Model file for the job. Use its own axes, mm. Face numbers are marked on the shaded views. Coordinates: 2 decimals unless noted, no trailing zeros. Write each loop counter-clockwise with the first axis right and the second up, starting at its lowest first coordinate (ties: lowest second). Pieces come first, ordered by that corner, then holes. Notation, with made-up numbers: M -32,74 L 24,74 A18 ccw 24,83 Z; hole C 13,83 d7. An arc over 180 degrees is marked long. Use CSV: the item, a comma, the result in double quotes. Start each with the question number.
from build123d import *

# Parameters (mm, degrees)
SKETCH1_W              = 22.5552
SKETCH1_H              = 12.7
BOSS_EXTRUDE1_DEPTH    = 1
SKETCH2_W              = 5
SKETCH2_H              = 7.3
CUT_EXTRUDE1_DEPTH     = 1
SKETCH3_W              = 5
SKETCH3_H              = 5
CUT_EXTRUDE2_DEPTH     = 1
SKETCH4_W              = 22.0552
SKETCH4_H              = 0.5
SKETCH4_W_2            = 0.5
SKETCH4_H_2            = 1.5
SKETCH4_H_3            = 2
BOSS_EXTRUDE2_DEPTH    = 1
SKETCH5_W              = 39.7552
SKETCH5_H              = 16.7
BOSS_EXTRUDE3_DEPTH    = 1
CUT_EXTRUDE3_DEPTH     = 1
CUT_EXTRUDE4_DEPTH     = 1
CUT_EXTRUDE5_START     = -4
CUT_EXTRUDE5_DEPTH     = 5
SKETCH10_W             = 22.5552
SKETCH10_H             = 2
BOSS_EXTRUDE4_DEPTH    = 2
SKETCH11_W             = 8.919893548
SKETCH11_H             = 0.730490532
CUT_EXTRUDE6_DEPTH     = 3
SKETCH12_W             = 22.5552
SKETCH12_H             = 1.5
BOSS_EXTRUDE5_DEPTH    = 2
SKETCH13_W             = 3
SKETCH13_H             = 1.5
CUT_EXTRUDE7_DEPTH     = 2
SKETCH14_W             = 2.125
SKETCH14_H             = 1.226869322
CUT_EXTRUDE8_DEPTH     = 1
SKETCH15_W             = 1.65
SKETCH15_H             = 11.12
ADAPTER_PCB_HOLE_DEPTH = 1
CUT_EXTRUDE10_DEPTH    = 1


with BuildPart() as part:
    # Sketch1 → Boss-Extrude1 (new body)
    with BuildSketch(Plane(origin=(0, 0, 0), x_dir=(1, 0, 0), z_dir=(0, 1, 0))):
        with Locations((-28.763088774, 14.606547542)):
            Rectangle(SKETCH1_W, SKETCH1_H)
    extrude(amount=BOSS_EXTRUDE1_DEPTH)

    # Sketch2 → Cut-Extrude1 (cut)
    with BuildSketch(Plane(origin=(0, 1, 0), x_dir=(1, 0, 0), z_dir=(0, 1, 0))):
        with Locations((-37.540688774, 14.606547542)):
            Rectangle(SKETCH2_W, SKETCH2_H)
    extrude(amount=-CUT_EXTRUDE1_DEPTH, mode=Mode.SUBTRACT)

    # Sketch3 → Cut-Extrude2 (cut)
    with BuildSketch(Plane(origin=(0, 1, 0), x_dir=(1, 0, 0), z_dir=(0, 1, 0))):
        with Locations((-19.985488774, 13.756547542)):
            Rectangle(SKETCH3_W, SKETCH3_H)
    extrude(amount=-CUT_EXTRUDE2_DEPTH, mode=Mode.SUBTRACT)

    # Sketch4 → Boss-Extrude2 (add)
    with BuildSketch(Plane.XZ):
        with Locations((-29.013088774, -8.506547542)):
            Rectangle(SKETCH4_W, SKETCH4_H)
        with Locations((-17.735488774, -8.506547542)):
            Rectangle(SKETCH4_W_2, SKETCH4_H)
        with Locations((-17.735488774, -9.506547542)):
            Rectangle(SKETCH4_W_2, SKETCH4_H_2)
        with Locations((-29.013088774, -20.706547542)):
            Rectangle(SKETCH4_W, SKETCH4_H)
        with Locations((-17.735488774, -19.456547542)):
            Rectangle(SKETCH4_W_2, SKETCH4_H_3)
        with Locations((-17.735488774, -20.706547542)):
            Rectangle(SKETCH4_W_2, SKETCH4_H)
    extrude(amount=BOSS_EXTRUDE2_DEPTH)

    # Sketch5 → Boss-Extrude3 (add)
    with BuildSketch(Plane(origin=(0, 1, 0), x_dir=(1, 0, 0), z_dir=(0, 1, 0))):
        with Locations((-33.363088774, 14.606547542)):
            Rectangle(SKETCH5_W, SKETCH5_H)
    extrude(amount=BOSS_EXTRUDE3_DEPTH)

    # Sketch6 → Cut-Extrude3 (cut)
    with BuildSketch(Plane(origin=(0, 2, 0), x_dir=(1, 0, 0), z_dir=(0, 1, 0))):
        Polygon((-39.790688774, 13.37967822), (-37.665688774, 12.152808898), (-35.540688774, 13.37967822), (-35.540688774, 15.833416864), (-37.665688774, 17.060286186), (-39.790688774, 15.833416864), align=None)
    extrude(amount=-CUT_EXTRUDE3_DEPTH, mode=Mode.SUBTRACT)

    # Sketch7 → Cut-Extrude4 (cut)
    with BuildSketch(Plane(origin=(0, 1, 0), x_dir=(-1, 0, 0), z_dir=(0, -1, 0))):
        Polygon((17.735488774, 14.983416864), (15.610488774, 16.210286186), (13.485488774, 14.983416864), (13.485488774, 12.52967822), (15.610488774, 11.302808898), (17.735488774, 12.52967822), align=None)
    extrude(amount=-CUT_EXTRUDE4_DEPTH, mode=Mode.SUBTRACT)

    # Sketch8 → Cut-Extrude5 (cut)
    with BuildSketch(Plane(origin=(0, 2, 0), x_dir=(1, 0, 0), z_dir=(0, 1, 0)).offset(CUT_EXTRUDE5_START)):
        with BuildLine():
            Line((-13.485488774, 22.956547542), (-22.127760886, 22.956547542))
            add(Edge.make_bspline(
                [(-22.127760886, 22.956547542), (-17.367981555, 22.956547542), (-14.30272025, 21.87197064), (-13.485488774, 18.176213027)],
                knots=[0, 0, 0, 0, 1, 1, 1, 1], degree=3))
            Line((-13.485488774, 18.176213027), (-13.485488774, 22.956547542))
        make_face()
    cut_extrude5 = extrude(amount=CUT_EXTRUDE5_DEPTH, mode=Mode.SUBTRACT)

    # Mirror2: Cut-Extrude5 across plane
    add(cut_extrude5.mirror(Plane.XY.offset(-14.61)), mode=Mode.SUBTRACT)

    # Sketch10 → Boss-Extrude4 (add)
    with BuildSketch(Plane(origin=(0, 1, 0), x_dir=(-1, 0, 0), z_dir=(0, -1, 0))):
        with Locations((28.763088774, 7.256547542)):
            Rectangle(SKETCH10_W, SKETCH10_H)
        with Locations((28.763088774, 21.956547542)):
            Rectangle(SKETCH10_W, SKETCH10_H)
    extrude(amount=BOSS_EXTRUDE4_DEPTH)

    # Sketch11 → Cut-Extrude6 (cut)
    with BuildSketch(Plane(origin=(0, 2, 0), x_dir=(1, 0, 0), z_dir=(0, 1, 0))):
        with Locations((-17.667814112, 5.898207192)):
            Rectangle(SKETCH11_W, SKETCH11_H)
    extrude(amount=-CUT_EXTRUDE6_DEPTH, mode=Mode.SUBTRACT)

    # Sketch12 → Boss-Extrude5 (add)
    with BuildSketch(Plane(origin=(0, -1, 0), x_dir=(-1, 0, 0), z_dir=(0, -1, 0))):
        with Locations((28.763088774, 7.006547542)):
            Rectangle(SKETCH12_W, SKETCH12_H)
        with Locations((28.763088774, 22.206547542)):
            Rectangle(SKETCH12_W, SKETCH12_H)
    extrude(amount=BOSS_EXTRUDE5_DEPTH)

    # Sketch13 → Cut-Extrude7 (cut)
    with BuildSketch(Plane(origin=(0, -3, 0), x_dir=(-1, 0, 0), z_dir=(0, -1, 0))):
        with Locations((35.040688774, 7.006547542)):
            Rectangle(SKETCH13_W, SKETCH13_H)
        with Locations((35.040688774, 22.206547542)):
            Rectangle(SKETCH13_W, SKETCH13_H)
        with Locations((22.040688774, 7.006547542)):
            Rectangle(SKETCH13_W, SKETCH13_H)
        with Locations((22.040688774, 22.206547542)):
            Rectangle(SKETCH13_W, SKETCH13_H)
    extrude(amount=-CUT_EXTRUDE7_DEPTH, mode=Mode.SUBTRACT)

    # Sketch14 → Cut-Extrude8 (cut)
    with BuildSketch(Plane(origin=(0, 2, 0), x_dir=(1, 0, 0), z_dir=(0, 1, 0))):
        with Locations((-14.547988774, 15.596851525)):
            Rectangle(SKETCH14_W, SKETCH14_H)
        with Locations((-14.547988774, 11.916243559)):
            Rectangle(SKETCH14_W, SKETCH14_H)
    extrude(amount=-CUT_EXTRUDE8_DEPTH, mode=Mode.SUBTRACT)

    # Sketch15 → adapter_PCB_hole (cut)
    with BuildSketch(Plane(origin=(0, 1, 0), x_dir=(-1, 0, 0), z_dir=(0, -1, 0))):
        with Locations((45.085688774, 14.606547542)):
            Rectangle(SKETCH15_W, SKETCH15_H)
    extrude(amount=-ADAPTER_PCB_HOLE_DEPTH, mode=Mode.SUBTRACT)

    # Sketch22 → Cut-Extrude10 (cut)
    with BuildSketch(Plane(origin=(0, 1, 0), x_dir=(-1, 0, 0), z_dir=(0, -1, 0))):
        Polygon((52.265688774, 15.836869322), (50.140688774, 17.063738644), (48.015688774, 15.836869322), (48.015688774, 13.383130678), (50.140688774, 12.156261356), (52.265688774, 13.383130678), align=None)
    extrude(amount=-CUT_EXTRUDE10_DEPTH, mode=Mode.SUBTRACT)


solid = part.part
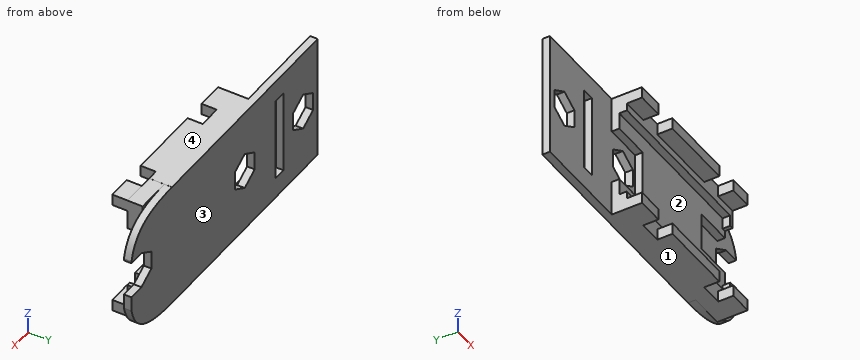
1) Band-saw the part on A-A on z = -14.25. List the corners of the cut face in (x, y), then the cut area to 3 significant figures.
2) Wall check: L1, parallel to Z at x = -31.5, y = -2.6; L2, parallel to Z at x = -39.5, y = -0.9; L3, parallel to X at y = 1.45, z = -17.5. Give the ranges that are in metal, low to high. Write a range as [from, to].
3) Two-plate mould, pull along Z, no slides. Class the marked faces 1, 2, 3 and 4: pulls with the +Z half, pulls with the -Z half, needs draft (parallel to the pull), parting line crosses it, or undercut.
4) Drop flat-ended pins along their axis: P1, Ø0.8, axis at x = -14.5, y = 1.5, coming from the +Z side; P2, Ø0.6, axis at x = -19, y = -0.5, coming from the +Z side; P3, Ø1, axis at y = -1, z = -17, coming from the -X side; P4, Ø1.6, axis at y = -2.5, z = -22, coming from the -X side. Give the stop position or say it passes through.
5) Band-saw the part on D-D on x = -43. List the corners of the cut face in (y, z), then the cut area to 3 significant figures.
6) Band-saw the part on B-B on x = -24.5. List the corners of the cut face in (y, z), then the cut area to 3 significant figures.
Findings below:
1,outline,"M -53.24,1 L -52.27,1 L -52.27,2 L -53.24,2 Z; M -48.02,1 L -45.91,1 L -45.91,2 L -48.02,2 Z; M -44.26,1 L -39.79,1 L -39.79,2 L -44.26,2 Z; M -35.54,1 L -35.04,1 L -35.04,0 L -22.49,0 L -22.49,1 L -17.74,1 L -17.74,2 L -35.54,2 Z"
1,area,"37.9 mm2"
2,L1,"z = [-22.96, -21.46], [-7.76, -6.26]"
2,L2,"z = [-22.96, -20.46], [-8.76, -6.26]"
2,L3,"x = [-53.24, -45.91], [-44.26, -13.49]"
3,face 1,"pulls with the -Z half"
3,face 2,"undercut"
3,face 3,"needs draft"
3,face 4,"pulls with the +Z half"
4,P1,"stops at z = -8.29"
4,P2,"stops at z = -6.26"
4,P3,"passes through"
4,P4,"stops at x = -40.04"
5,outline,"M 1,-22.96 L 2,-22.96 L 2,-6.26 L 1,-6.26 Z"
5,area,"16.7 mm2"
6,outline,"M -3,-22.96 L 2,-22.96 L 2,-6.26 L -3,-6.26 L -3,-7.76 L -1,-7.76 L -1,-8.76 L 0,-8.76 L 0,-20.46 L -1,-20.46 L -1,-21.46 L -3,-21.46 Z"
6,area,"44.4 mm2"
